For this review, take the finished solid that the model builds, in its own axes (mm). A direction names the side the tool comes from. Give positions to 0.01 mm unless a question says otherwise; leave off trailing zeros. Loops run counter-clockwise (first coordinate to the right, second up) from the corner with the lowest first, then second, coordinate; pieces in that order, holes last. Notation, with made-up numbers: (-27, 68) - (-6, 68) arc R32 ccw to (-6, 96) - close; hole circle Ø2 at (8.25, 0). An arc over 180 degrees is marked (long way). Answer in a Markdown table with one row per item.
```python
from build123d import *

# Parameters (mm, degrees)
SKETCH_1_R      = 1.5
SKETCH_1_W      = 38
SKETCH_1_H      = 50
EXTRUDE_1_DEPTH = 4


with BuildPart() as part:
    # 草图1 → 凸台-拉伸1 (new body)
    with BuildSketch(Plane(origin=(0, 0, 0), x_dir=(1, 0, 0), z_dir=(0, 1, 0))):
        Polygon((-12, 48.5), (-12, 32.5), (12, 32.5), (12, 48.5), (42.5, 48.5), (42.5, -48.5), (12, -48.5), (12, -32.5), (-12, -32.5), (-12, -48.5), (-42.5, -48.5), (-42.5, 48.5), align=None)
        with Locations(Location((15, 41.5, 0), (0, 0, 270))):
            Circle(SKETCH_1_R, mode=Mode.SUBTRACT)
        with Locations(Location((25, 41.5, 0), (0, 0, 270))):
            Circle(SKETCH_1_R, mode=Mode.SUBTRACT)
        with Locations(Location((-25, 41.5, 0), (0, 0, 90))):
            Circle(SKETCH_1_R, mode=Mode.SUBTRACT)
        with Locations(Location((-15, 41.5, 0), (0, 0, 90))):
            Circle(SKETCH_1_R, mode=Mode.SUBTRACT)
        with Locations(Location((25, -41.5, 0), (0, 0, 90))):
            Circle(SKETCH_1_R, mode=Mode.SUBTRACT)
        with Locations(Location((15, -41.5, 0), (0, 0, 90))):
            Circle(SKETCH_1_R, mode=Mode.SUBTRACT)
        with Locations(Location((-15, -41.5, 0), (0, 0, 270))):
            Circle(SKETCH_1_R, mode=Mode.SUBTRACT)
        with Locations(Location((-25, -41.5, 0), (0, 0, 270))):
            Circle(SKETCH_1_R, mode=Mode.SUBTRACT)
        Rectangle(SKETCH_1_W, SKETCH_1_H, mode=Mode.SUBTRACT)
    extrude(amount=EXTRUDE_1_DEPTH)


solid = part.part
```
1. Wall thickness on line 1 (X direction, y = 3.25, z = -41.5); line 2 (Z direction, x = 1, y = 2.7); line 3 (X direction, y = 0.9, z = -14.5): over which ranges is each line inside the solid? List them lowest first. Write a range as [from, to].
Values:
| item | result |
|---|---|
| line 1 | x = [-42.5, -26.5], [-23.5, -16.5], [-13.5, -12], [12, 13.5], [16.5, 23.5], [26.5, 42.5] |
| line 2 | z = [-32.5, -25], [25, 32.5] |
| line 3 | x = [-42.5, -19], [19, 42.5] |
2. Mouldability with a two-part tool opening along X and no side actions: class faces 1 (the face through (-15, 2, -40)), 2 (the face through (-27, 2, -48.5)), 3 (the face through (0, 2, 25)) as released by +X, released by -X, zero draft, split by the parting line, or undercut.
Values:
| item | result |
|---|---|
| face 1 | undercut |
| face 2 | zero draft |
| face 3 | undercut |
3. We need section D-D, the plane z = -41.5. Give the boundary of the cut face in (x, y), and give its area (3 significant figures).
Values:
| item | result |
|---|---|
| outline | (-42.5, 0) - (-26.5, 0) - (-26.5, 4) - (-42.5, 4) - close; (-23.5, 0) - (-16.5, 0) - (-16.5, 4) - (-23.5, 4) - close; (-13.5, 0) - (-12, 0) - (-12, 4) - (-13.5, 4) - close; (12, 0) - (13.5, 0) - (13.5, 4) - (12, 4) - close; (16.5, 0) - (23.5, 0) - (23.5, 4) - (16.5, 4) - close; (26.5, 0) - (42.5, 0) - (42.5, 4) - (26.5, 4) - close |
| area | 196 mm^2 |
4. Clearance check with flat-ended pins moving along their axes: pin 1 (1.5 mm diameter, centred on x = 4.5, y = 1.5, fed in from +Z); pin 2 (2.5 mm diameter, centred on x = -15, z = -41.5, fed in from -Y). State where each tip first meets the part, or that it passes through.
Values:
| item | result |
|---|---|
| pin 1 | stops at z = 32.5 |
| pin 2 | passes through |
5. For faces 4 (the face through (-19, 2, 0)), 5 (the face through (-27, 2, 48.5)), 6 (the face through (0, 2, 32.5)), list the 3-axis set-ups (+Z, -Z, +X, -X, +Y, -Y) from which the entire face can be reached by the end or side of a thin tool; tool diameter is ignored.
Values:
| item | result |
|---|---|
| face 4 | +Y, -Y |
| face 5 | +Z, +X, -X, +Y, -Y |
| face 6 | +Z, +Y, -Y |
6. We need section B-B, the plane x = 5.5. Give the boundary of the cut face in (y, z), and give its area (3 significant figures).
Values:
| item | result |
|---|---|
| outline | (0, -32.5) - (4, -32.5) - (4, -25) - (0, -25) - close; (0, 25) - (4, 25) - (4, 32.5) - (0, 32.5) - close |
| area | 60.0 mm^2 |
7. We need section C-C, the plane y = 3.1. Count the separate pieces of the cut face and the enclosed holes in it, and give its area (3 significant figures).
Values:
| item | result |
|---|---|
| separate pieces | 1 |
| enclosed holes | 9 |
| area | 5,520 mm^2 |
8. We need section A-A, the plane x = 25. Give the boundary of the cut face in (y, z).
Values:
| item | result |
|---|---|
| outline | (0, -48.5) - (4, -48.5) - (4, -43) - (0, -43) - close; (0, -40) - (4, -40) - (4, 40) - (0, 40) - close; (0, 43) - (4, 43) - (4, 48.5) - (0, 48.5) - close |
